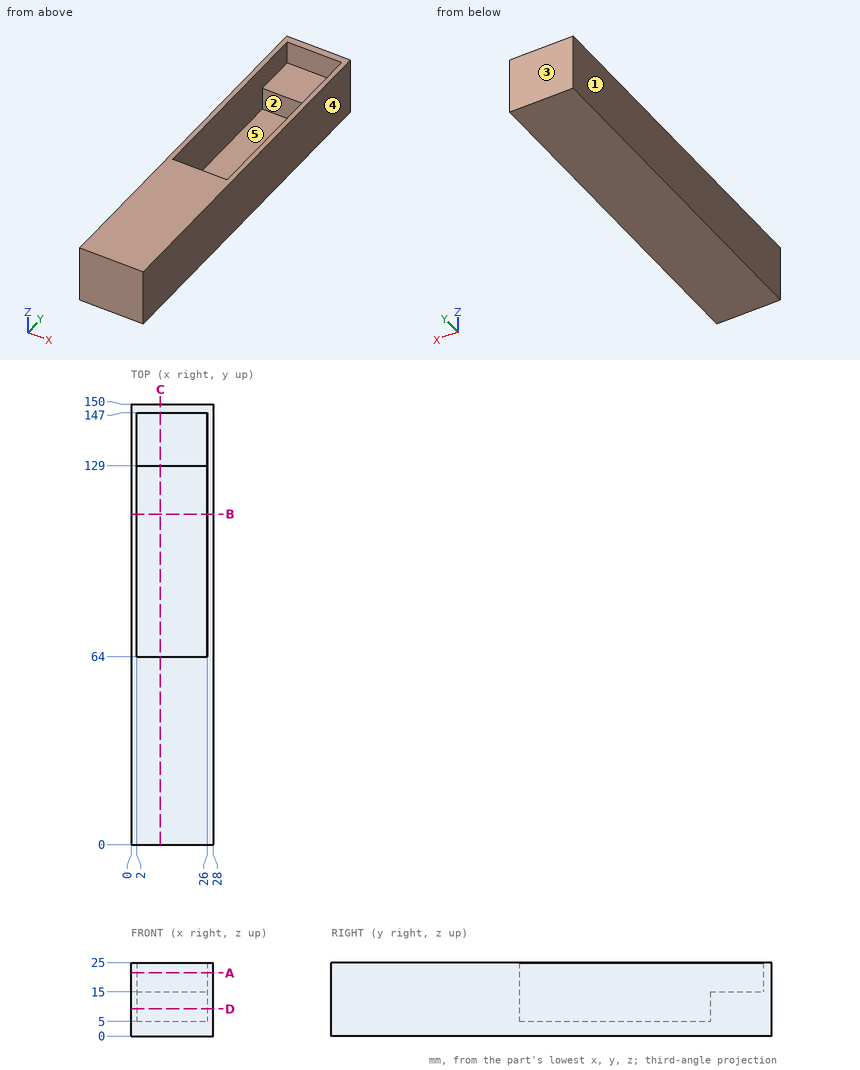
Study the drawing (mm; zero at the part's minimum x, y, z) and answer. A direction names the side the tool comes from. Round coordinates to 2 decimals unless told otherwise and drop trailing zeros. Write each loop counter-clockwise with the first axis right and the second up, starting at its lowest first coordinate (ties: lowest second). Pieces come first, ordered by that corner, then holes. Notation, with made-up numbers: (59, 60.25) - (81, 60.25) arc R26 cw to (81, 77.25) - close; hole circle Ø9 at (15.5, -23). An arc over 180 degrees is marked (long way). Return JSON: item names as keys, results as strings. Group by question number.
Q1. Find the intervals of material crossed by L1, parallel to Y at x = 13.25, z = 18; L2, parallel to Y at x = 8.75, z = 8.5; L3, parallel to X at y = 91.5, z = 14.25, in increasing order.
Q2. Each of these flat-tipped pins is pushed along its axis until it touches: pin 1 Ø9 at (x, y) = (13.5, 140) entering from +Z; pin 2 Ø3 at (x, y) = (15, 70.5) entering from +Z. Where does it stop, or does it pass through?
Q3. The part is cut by section D-D on z = 9.25. Write down the section's boundary in (x, y), then the cut area to 3 significant figures.
Q4. The part is cut by section B-B on y = 112.5. Write down the section's boundary in (x, z).
Q5. The mould has two halves that part along X. Classify the marked faces 3, 4 and 5: released by +X, released by -X, zero draft, split by the parting line, or undercut.
Q6. The part is cut by section A-A on z = 21.5. Write down the section's boundary in (x, y).
Q7. The part is cut by section C-C on x = 10. Write down the section's boundary in (y, z).
Q8. For the marked faces 1 and 2, determine the directions among +Z, -Z, +X, -X, +Y, -Y from which every point of the face is accessible in a straight line to the end or side of a thin tool.
Solved:
{
 "1": {"L1": "0 to 64, 147 to 150", "L2": "0 to 64, 129 to 150", "L3": "0 to 2, 26 to 28"},
 "2": {"pin 1": "z = 15", "pin 2": "z = 5"},
 "3": {"outline": "(0, 0) - (28, 0) - (28, 150) - (0, 150) - close; hole (2, 64) - (26, 64) - (26, 129) - (2, 129) - close", "area": "2,640 mm²"},
 "4": {"outline": "(0, 0) - (28, 0) - (28, 25) - (26, 25) - (26, 5) - (2, 5) - (2, 25) - (0, 25) - close"},
 "5": {"face 3": "zero draft", "face 4": "released by +X", "face 5": "undercut"},
 "6": {"outline": "(0, 0) - (28, 0) - (28, 150) - (0, 150) - close; hole (2, 64) - (26, 64) - (26, 147) - (2, 147) - close"},
 "7": {"outline": "(0, 0) - (150, 0) - (150, 25) - (147, 25) - (147, 15) - (129, 15) - (129, 5) - (64, 5) - (64, 25) - (0, 25) - close"},
 "8": {"face 1": "+Z, -Z, -X, +Y, -Y", "face 2": "+Z"}
}
